Design review of the part built by this model. Coordinates are the model's own, in mm. Round coordinates to 2 decimals unless told otherwise and drop trailing zeros. Loops run counter-clockwise (first coordinate to the right, second up) from the corner with the lowest first, then second, coordinate; pieces in that order, holes last. Notation, with made-up numbers: M 66,10 L 83,10 A17 cw 83,24 Z; hole C 17.5,52 d11. An arc over 180 degrees is marked long. Answer as CSV lines item,"result". Start each with the question number.
from build123d import *

# Parameters (mm, degrees)
SKETCH2_R           = 5
BOSS_EXTRUDE1_DEPTH = 10
FILLET1_R           = 3
BOSS_EXTRUDE2_DEPTH = 10
SKETCH5_R           = 5
SKETCH5_R_2         = 4.5
BOSS_EXTRUDE3_DEPTH = 10
SKETCH6_R           = 2
CUT_EXTRUDE1_DEPTH  = 10
SKETCH7_R           = 3
CUT_EXTRUDE2_DEPTH  = 10


with BuildPart() as part:
    # Sketch2 → Boss-Extrude1 (new body)
    with BuildSketch(Plane(origin=(0, 0, 0), x_dir=(1, 0, 0), z_dir=(0, 1, 0))):
        with BuildLine():
            Line((36.25, 10), (-36.25, 10))
            ThreePointArc((-36.25, 10), (-46.25, 0), (-36.25, -10))
            Line((-36.25, -10), (36.25, -10))
            ThreePointArc((36.25, -10), (46.25, 0), (36.25, 10))
        make_face()
        with Locations((-36.25, 0)):
            Circle(SKETCH2_R, mode=Mode.SUBTRACT)
        with BuildLine():
            ThreePointArc((5, 0), (3.535533906, -3.535533906), (0, -5))
            ThreePointArc((0, -5), (-5, 0), (0, 5))
            ThreePointArc((0, 5), (3.535533906, 3.535533906), (5, 0))
        make_face(mode=Mode.SUBTRACT)
        with Locations((36.25, 0)):
            Circle(SKETCH2_R, mode=Mode.SUBTRACT)
    extrude(amount=BOSS_EXTRUDE1_DEPTH)

    # Fillet1
    fillet1_edges = [part.edges().sort_by_distance(p)[0] for p in [
        (46.25, 0, 0),
        (0, 0, 10),
        (0, 10, 10),
        (46.25, 10, 0),
        (0, 10, -10),
        (-46.25, 10, 0),
        (-46.25, 0, 0),
        (0, 0, -10),
    ]]
    fillet(fillet1_edges, radius=FILLET1_R)

    # Sketch3 → Boss-Extrude2 (add)
    with BuildSketch(Plane(origin=(0, 10, 0), x_dir=(1, 0, 0), z_dir=(0, 1, 0))):
        with BuildLine():
            Line((5, 0), (0, 0))
            Line((0, 0), (-5, 0))
            ThreePointArc((-5, 0), (0, -5), (5, 0))
        make_face()
        with BuildLine():
            Line((-5, 0), (0, 0))
            Line((0, 0), (5, 0))
            ThreePointArc((5, 0), (0, 5), (-5, 0))
        make_face()
    extrude(amount=-BOSS_EXTRUDE2_DEPTH)

    # Sketch5 → Boss-Extrude3 (add)
    with BuildSketch(Plane(origin=(0, 10, 0), x_dir=(1, 0, 0), z_dir=(0, 1, 0))):
        with Locations((-36.25, 0)):
            Circle(SKETCH5_R)
        with Locations((-36.25, 0)):
            Circle(SKETCH5_R_2, mode=Mode.SUBTRACT)
        with Locations((36.25, 0)):
            Circle(SKETCH5_R)
        with Locations((36.25, 0)):
            Circle(SKETCH5_R_2, mode=Mode.SUBTRACT)
    extrude(amount=-BOSS_EXTRUDE3_DEPTH)

    # Sketch6 → Cut-Extrude1 (cut)
    with BuildSketch(Plane(origin=(0, 10, 0), x_dir=(1, 0, 0), z_dir=(0, 1, 0))):
        with Locations((-7, 0)):
            Circle(SKETCH6_R)
        with Locations((7, 0)):
            Circle(SKETCH6_R)
    extrude(amount=-CUT_EXTRUDE1_DEPTH, mode=Mode.SUBTRACT)

    # Sketch7 → Cut-Extrude2 (cut)
    with BuildSketch(Plane(origin=(0, 10, 0), x_dir=(1, 0, 0), z_dir=(0, 1, 0))):
        Circle(SKETCH7_R)
    extrude(amount=-CUT_EXTRUDE2_DEPTH, mode=Mode.SUBTRACT)


solid = part.part
Item 1: Consider section C-C, the plane z = 0. Write out the cut boundary in (x, y), then the cut area to 3 significant figures.
Item 2: Insertion check: pin 1 Ø7 at (x, z) = (36.25, 0) entering from -Y; pin 2 Ø1 at (y, z) = (2, 2.5) entering from +X; pin 3 Ø1 at (y, z) = (3.5, -6.5) entering from +X; pin 4 Ø6 at (y, z) = (4.5, -6.5) entering from -X. Each pin has a flat end and moves straight along its axis. Give the tip position at first contact, or say it passes through.
Item 3: Consider section D-D, the plane x = -21. Write out the cut boundary in (y, z), then the cut area to 3 significant figures.
Item 4: To check wall thickness, follow line 1 (X direction, y = 5, z = 0); line 2 (Z direction, x = -7, y = 3.25); line 3 (X direction, y = 8, z = 0). State the ranges of each line that lie inside material, in increasing order.
Item 5: Consider section B-B, the plane x = -7. Write out the cut boundary in (y, z).
Item 6: Consider section A-A, the plane y = 6. Write out the cut boundary in (x, z), then the cut area to 3 significant figures.
Item 7: The part is to be moulded in two halves that separate along X. For faces 1 (the face through (-46.248, 4.972, -0.22)), 2 (the face through (-3, 5, 0)), 3 (the face through (0.51, 0.9, 9.14)), 4 (the face through (46.248, 4.972, 0.22)), say which applies: +X half, -X half, draft (parallel to the pull), parting line (faces both ways), or undercut.
Found:
1,outline,"M -46.25,3 A3 ccw -43.25,0 L -40.75,0 L -40.75,10 L -43.25,10 A3 ccw -46.25,7 Z; M -31.75,0 L -9,0 L -9,10 L -31.75,10 Z; M -5,0 L -3,0 L -3,10 L -5,10 Z; M 3,0 L 5,0 L 5,10 L 3,10 Z; M 9,0 L 31.75,0 L 31.75,10 L 9,10 Z; M 40.75,0 L 43.25,0 A3 ccw 46.25,3 L 46.25,7 A3 ccw 43.25,10 L 40.75,10 Z"
1,area,"597 mm^2"
2,pin 1,"passes through"
2,pin 2,"stops at x = 45.94"
2,pin 3,"stops at x = 44.25"
2,pin 4,"stops at x = -45.62"
3,outline,"M 0,-7 A3 ccw 3,-10 L 7,-10 A3 ccw 10,-7 L 10,7 A3 ccw 7,10 L 3,10 A3 ccw 0,7 Z"
3,area,"192 mm^2"
4,line 1,"x = -46.25 to -40.75, -31.75 to -9, -5 to -3, 3 to 5, 9 to 31.75, 40.75 to 46.25"
4,line 2,"z = -10 to -2, 2 to 10"
4,line 3,"x = -46.08 to -40.75, -31.75 to -9, -5 to -3, 3 to 5, 9 to 31.75, 40.75 to 46.08"
5,outline,"M 0,-7 A3 ccw 3,-10 L 7,-10 A3 ccw 10,-7 L 10,-2 L 0,-2 Z; M 0,2 L 10,2 L 10,7 A3 ccw 7,10 L 3,10 A3 ccw 0,7 Z"
6,outline,"M -36.25,-10 L 36.25,-10 A10 ccw 36.25,10 L -36.25,10 A10 ccw Z; hole C -36.25,0 d9; hole C -7,0 d4; hole C 0,0 d6; hole C 7,0 d4; hole C 36.25,0 d9"
6,area,"1,580 mm^2"
7,face 1,"-X half"
7,face 2,"undercut"
7,face 3,"draft"
7,face 4,"+X half"
